```python
from build123d import *

# Parameters (mm, degrees)
F0_W     = 143.67862
F0_H     = 198.66103
F1_DEPTH = 5.08
F2_W     = 118.27862
F2_H     = 12.7
F2_W_2   = 25.4
F2_H_2   = 25.4
F3_DEPTH = 101.6


with BuildPart() as f1:
    # F0 (on Top) → F1 (new body)
    with BuildSketch(Plane.XY):
        Rectangle(F0_W, F0_H)
    extrude(amount=F1_DEPTH)

    # F2 (on face) → F3 (join)
    with BuildSketch(Plane.XY.offset(5.08)):
        Polygon((-59.13931, 99.330515), (-71.83931, 99.330515), (-71.83931, -99.330515), (-59.13931, -99.330515), (-59.13931, -73.930515), (-59.13931, 86.630515), align=None)
        with Locations((0, 92.980515)):
            Rectangle(F2_W, F2_H)
        Polygon((71.83931, 99.330515), (59.13931, 99.330515), (59.13931, 86.630515), (59.13931, -73.930515), (59.13931, -99.330515), (71.83931, -99.330515), align=None)
        with Locations((-46.43931, -86.630515)):
            Rectangle(F2_W_2, F2_H_2)
        with Locations((46.43931, -86.630515)):
            Rectangle(F2_W_2, F2_H_2)
    extrude(amount=F3_DEPTH)


solid = f1.part
```
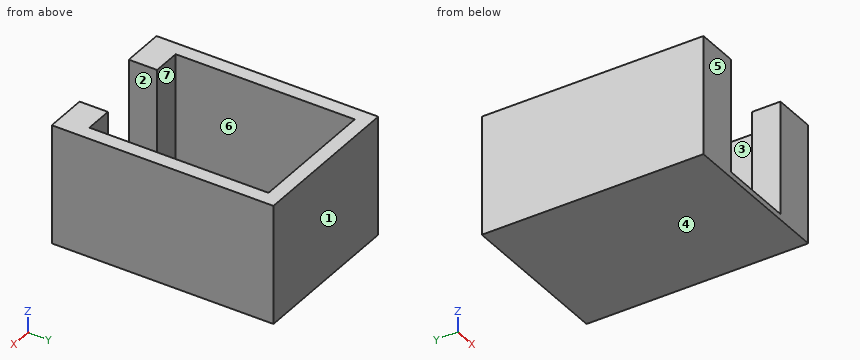
Part model, mm, in its own coordinate system. Face numbers are marked on the shaded views. A direction names the side the tool comes from. Coordinates: 2 decimals unless noted, no trailing zeros. Loops run counter-clockwise (first coordinate to the right, second up) from the corner with the lowest first, then second, coordinate; pieces in that order, holes last. Notation, with made-up numbers: (53.25, 26.25) - (110.25, 26.25) arc R13 ccw to (110.25, 39.25) - close; hole circle Ø7 at (-19.5, 10.25). An arc over 180 degrees is marked (long way). Write item = value, one per line. Start each with the question number.
Item 1: Cut at A-A, the plane z = 87.5. Give the cut face in (x, y).
Item 2: 3-axis set-ups, long thin cutter, end or side, ignore diameter. For the marked faces 1, 2 and 3: which of +Z, -Z, +X, -X, +Y, -Y reach the whole face in a straight line?
Item 3: Cut at D-D, the plane x = -55.5. Give the cut face in (y, z).
Item 4: Cut at B-B, the plane y = -33. Give the cut face in (x, z), and give its area (3 significant figures).
Item 5: Flat gauge pin, fed straight in: pin 1 Ø2 at (x, y) = (37.5, 18) entering from +Z. Where does the tip first touch, or does it go through?
Item 6: Wall check: L1, parallel to Y at x = 47, z = 12.5; L2, parallel to X at y = 6, z = 63; L3, parallel to Y at x = -33.5, z = 16.5. Give the ranges that are in metal, low to high. Write a range as from..to.
Item 7: Mould opens along Y. For the marked faces 4, 5, 6 and 7 say: released by +Y, released by -Y, zero draft, split by the parting line, or undercut.
Item 8: Cut at C-C, the plane x = 10. Give the cut face in (y, z).
The answers:
q1.outline = (-71.84, -99.33) - (-33.74, -99.33) - (-33.74, -73.93) - (-59.14, -73.93) - (-59.14, 86.63) - (59.14, 86.63) - (59.14, -73.93) - (33.74, -73.93) - (33.74, -99.33) - (71.84, -99.33) - (71.84, 99.33) - (-71.84, 99.33) - close
q2.face_1 = +Z, -Z, +X, -X, +Y
q2.face_2 = +Z, -Y
q2.face_3 = +Z
q3.outline = (-99.33, 0) - (99.33, 0) - (99.33, 106.68) - (86.63, 106.68) - (86.63, 5.08) - (-73.93, 5.08) - (-73.93, 106.68) - (-99.33, 106.68) - close
q4.outline = (-71.84, 0) - (71.84, 0) - (71.84, 106.68) - (59.14, 106.68) - (59.14, 5.08) - (-59.14, 5.08) - (-59.14, 106.68) - (-71.84, 106.68) - close
q4.area = 3,310 mm2
q5.pin_1 = 5.08
q6.L1 = -99.33..-73.93, 86.63..99.33
q6.L2 = -71.84..-59.14, 59.14..71.84
q6.L3 = 86.63..99.33
q7.face_4 = zero draft
q7.face_5 = released by -Y
q7.face_6 = undercut
q7.face_7 = undercut
q8.outline = (-99.33, 0) - (99.33, 0) - (99.33, 106.68) - (86.63, 106.68) - (86.63, 5.08) - (-99.33, 5.08) - close
